```python
from build123d import *

# Parameters (mm, degrees)
CUT_EXTRUDE1_DEPTH      = 21
CUT_EXTRUDE1_DEPTH_BACK = 22
SKETCH4_R               = 1.7
SKETCH5_R               = 1
CUT_EXTRUDE2_DEPTH      = 32
CUT_EXTRUDE3_DEPTH      = 106.948100502
CUT_EXTRUDE3_DEPTH_BACK = 61
SKETCH7_R               = 1.7
SKETCH8_R               = 1.7
CUT_EXTRUDE4_DEPTH      = 25
SKETCH9_R               = 1
CUT_EXTRUDE5_DEPTH      = 25
SKETCH10_R              = 4.5
CUT_EXTRUDE6_DEPTH      = 10
SKETCH11_R              = 3
CUT_EXTRUDE7_DEPTH      = 13


with BuildPart() as part:
    # Sketch1 → Revolve1 (revolve)
    with BuildSketch(Plane.XY, mode=Mode.PRIVATE) as revolve1_sk:
        Polygon((0, 0), (0, 24.820612545), (68.489462458, 24.820612545), (68.489462458, 22.028059354), (84.491973548, 22.028059354), (84.491973548, 25), (90, 25), (90, 0), align=None)
    revolve(revolve1_sk.sketch.rotate(Axis((0, 0, 0), (-1, 0, 0)), 90), axis=Axis((0, 0, 0), (-1, 0, 0)))

    # Sketch3 → Cut-Revolve1 (revolve, cut)
    with BuildSketch(Plane(origin=(0, 0, 0), x_dir=(1, 0, 0), z_dir=(0, 1, 0))):
        Polygon((0, 0), (0, 13), (11.186820081, 13), (11.186820081, 11), (14.393242315, 11), (14.393242315, 9), (69.922645544, 9), (69.922645544, 5), (81.873855688, 5), (81.873855688, 7), (90, 7), (90, 0), align=None)
    revolve(axis=Axis((96.448502204, 0, 0), (-1, 0, 0)), mode=Mode.SUBTRACT)

    # Sketch4 → Cut-Extrude1 (cut, two sides: drawn at the far end of the back side and taken through both)
    with BuildSketch(Plane.XY.offset(-CUT_EXTRUDE1_DEPTH_BACK)):
        with Locations(Location((38.043963981, 0, 0), (0, 0, 180))):
            Circle(SKETCH4_R)
    extrude(amount=CUT_EXTRUDE1_DEPTH + CUT_EXTRUDE1_DEPTH_BACK, mode=Mode.SUBTRACT)

    # Sketch5 → Cut-Extrude2 (cut)
    with BuildSketch(Plane.XY):
        with Locations((10.543963981, 0)):
            Circle(SKETCH5_R)
    extrude(amount=-CUT_EXTRUDE2_DEPTH, mode=Mode.SUBTRACT)

    # Sketch7 → Cut-Extrude3 (cut, two sides: drawn at the far end of the back side and taken through both)
    with BuildSketch(Plane(origin=(0, 25, 0), x_dir=(1, 0, 0), z_dir=(0, 1, 0)).offset(-CUT_EXTRUDE3_DEPTH_BACK)):
        with Locations(Location((37.989462458, 0, 0), (0, 0, 90))):
            Circle(SKETCH7_R)
    extrude(amount=CUT_EXTRUDE3_DEPTH + CUT_EXTRUDE3_DEPTH_BACK, mode=Mode.SUBTRACT)

    # Sketch8 → Cut-Extrude4 (cut)
    with BuildSketch(Plane.XY.offset(25)):
        with Locations((63.489462458, 0)):
            Circle(SKETCH8_R)
    extrude(amount=-CUT_EXTRUDE4_DEPTH, mode=Mode.SUBTRACT)

    # Sketch9 → Cut-Extrude5 (cut)
    with BuildSketch(Plane(origin=(0, 25, 0), x_dir=(1, 0, 0), z_dir=(0, 1, 0))):
        with Locations(Location((9.489462458, 0, 0), (0, 0, 270))):
            Circle(SKETCH9_R)
    extrude(amount=-CUT_EXTRUDE5_DEPTH, mode=Mode.SUBTRACT)

    # Sketch10 → Cut-Extrude6 (cut)
    with BuildSketch(Plane(origin=(0, 25, 0), x_dir=(1, 0, 0), z_dir=(0, 1, 0))):
        with Locations(Location((37.989462458, 0, 0), (0, 0, 270))):
            Circle(SKETCH10_R)
    cut_extrude6 = extrude(amount=-CUT_EXTRUDE6_DEPTH, mode=Mode.SUBTRACT)

    # Mirror1: Cut-Extrude6 across plane
    add(cut_extrude6.mirror(Plane.ZX), mode=Mode.SUBTRACT)

    # Sketch11 → Cut-Extrude7 (cut)
    with BuildSketch(Plane.XY.offset(25)):
        with Locations((63.489462458, 0)):
            Circle(SKETCH11_R)
    extrude(amount=-CUT_EXTRUDE7_DEPTH, mode=Mode.SUBTRACT)


solid = part.part
```
Source: CAD feature listing. Evaluate the final solid. Frame: model axes, mm. A direction names the side the tool comes from. Coordinates: 2 decimals unless noted, no trailing zeros. Loops run counter-clockwise (first coordinate to the right, second up) from the corner with the lowest first, then second, coordinate; pieces in that order, holes last. Notation, with made-up numbers: (-2.5, 84) - (33.5, 84) arc R21 ccw to (33.5, 107) - close; hole circle Ø7 at (74, 87.25). An arc over 180 degrees is marked (long way). Answer as CSV lines item,"result".
1. Section A-A (z = 10). Return loops of the section in (x, y).
Established:
outline,"(0, -22.72) - (68.49, -22.72) - (68.49, -19.63) - (84.49, -19.63) - (84.49, -22.91) - (90, -22.91) - (90, 22.91) - (84.49, 22.91) - (84.49, 19.63) - (68.49, 19.63) - (68.49, 22.72) - (0, 22.72) - (0, 8.31) - (11.19, 8.31) - (11.19, 4.58) - (14.39, 4.58) - (14.39, -4.58) - (11.19, -4.58) - (11.19, -8.31) - (0, -8.31) - close; hole circle Ø3.4 at (38.04, 0); hole circle Ø3.4 at (63.49, 0)"
2. Reachability of faces 1 (the flat face through (63, -2, 12)), 2 (the flat face through (84.492, 22.11, 1.74)), 3 (the cylindrical face through (11.47, -0.38, -17.8)), 4 (the cylindrical face through (85.994, 2.681, -6.466)), 5 (the cylindrical face through (42.547, -8.923, 1.172)) from +Z, -Z, +X, -X, +Y, -Y: full face, straight path, thin tool, end or side. Return the list, or none.
Established:
face 1,"+Z"
face 2,"none"
face 3,"-Z"
face 4,"+X"
face 5,"-X"
3. Section B-B (z = 0). Count the separate pieces of the cut face and the enclosed holes in it, then the cut area to 3 significant figures.
Established:
separate pieces,"5"
enclosed holes,"0"
area,"2,540 mm2"
4. Section D-D (x = 7). Return loops of the section in (y, z).
Established:
outline,"circle Ø49.64 at (0, 0); hole circle Ø26 at (0, 0)"
5. Contact query for flat-ended pins moving along their axis: pin 1 (1 mm diameter, centred on x = 29, y = 11.5, fed in from -Z); pin 2 (10 mm diameter, centred on x = 38.5, z = -1, fed in from +Y); pin 3 (11.5 mm diameter, centred on y = 0, z = 0, fed in from -X). Output: stop coordinate, or through.
Established:
pin 1,"stops at z = -22.25"
pin 2,"stops at y = 24.82"
pin 3,"stops at x = 69.92"
6. Section C-C (y = 20). Return loops of the section in (x, z).
Established:
outline,"(0, -14.7) - (68.49, -14.7) - (68.49, -9.23) - (84.49, -9.23) - (84.49, -15) - (90, -15) - (90, 15) - (84.49, 15) - (84.49, 9.23) - (68.49, 9.23) - (68.49, 14.7) - (0, 14.7) - close; hole circle Ø2 at (9.49, 0); hole circle Ø9 at (37.99, 0)"
7. Mould query, pull axis X, two halves, no side actions, for faces 6 (the flat face through (90, 5.2, -5.2)), 7 (the flat face through (0, 11, 11)), 8 (the cylindrical face through (42.45, -19.99, -0.59)). Classes: released by +X, released by -X, zero draft, split by the parting line, or undercut.
Established:
face 6,"released by +X"
face 7,"released by -X"
face 8,"undercut"
8. Ray query, line 1 (Y direction, x = 86.75, z = 0); line 2 (X direction, y = -12, z = 0); line 3 (X direction, y = -4.5, z = 3). Return the intervals inside material, ascending.
Established:
line 1,"y = -25 to -7, 7 to 25"
line 2,"x = 11.19 to 36.29, 39.69 to 90"
line 3,"x = 69.92 to 81.87"
